from build123d import *

# Parameters (mm, degrees)
SKETCH1_R           = 42.8625
SKETCH1_R_2         = 11.1125
BOSS_EXTRUDE1_DEPTH = 9.525
SKETCH2_R           = 7.9375
CUT_EXTRUDE1_DEPTH  = 10.16
SKETCH3_W           = 3.683
SKETCH3_H           = 25.4
CUT_EXTRUDE2_DEPTH  = 3.429
DRAFT2_ANGLE        = -2.5


with BuildPart() as part:
    # Sketch1 → Boss-Extrude1 (new body, symmetric)
    with BuildSketch(Plane.XY):
        Circle(SKETCH1_R)
        with Locations((0, 24.13)):
            Circle(SKETCH1_R_2, mode=Mode.SUBTRACT)
        with Locations((-20.897192993, -12.065)):
            Circle(SKETCH1_R_2, mode=Mode.SUBTRACT)
        with Locations((20.897192993, -12.065)):
            Circle(SKETCH1_R_2, mode=Mode.SUBTRACT)
    extrude(amount=BOSS_EXTRUDE1_DEPTH, both=True)

    # Sketch2 → Cut-Extrude1 (cut)
    with BuildSketch(Plane.XY.offset(9.525)):
        Circle(SKETCH2_R)
    extrude(amount=-CUT_EXTRUDE1_DEPTH, mode=Mode.SUBTRACT)

    # Sketch3 → Cut-Extrude2 (cut)
    with BuildSketch(Plane.XY.offset(9.525)):
        with Locations((0, -1.27)):
            Rectangle(SKETCH3_W, SKETCH3_H)
    extrude(amount=-CUT_EXTRUDE2_DEPTH, mode=Mode.SUBTRACT)

    # Draft2
    draft2_faces = [part.faces().sort_by_distance(p)[0] for p in [
        (-32.009692993, -12.065, 0),
        (9.784692993, -12.065, 0),
        (-11.1125, 24.13, 0),
    ]]
    draft(draft2_faces, Plane(origin=(0, 0, -9.525), x_dir=(-1, 0, 0), z_dir=(0, 0, -1)), DRAFT2_ANGLE)


solid = part.part
Check sheet for the modelled part. Datum: model origin and axes. Units: mm. A direction names the side the tool comes from. Coordinates: 2 decimals unless noted, no trailing zeros. Loops run counter-clockwise (first coordinate to the right, second up) from the corner with the lowest first, then second, coordinate; pieces in that order, holes last. Notation, with made-up numbers: (70.25, 22.25) -> (99.25, 22.25) arc R21 ccw to (99.25, 58.25) -> close; hole circle Ø9 at (-30.75, -9). An arc over 180 degrees is marked (long way). Answer in a Markdown table with one row per item.
1. Sectioned sample at C-C, the plane x = 0. Record the boundary of the cut face in (y, z) (1 decimal).
Check values:
| item | result |
|---|---|
| outline | (-42.9, -9.5) -> (13, -9.5) -> (12.2, 9.5) -> (11.4, 9.5) -> (11.4, 6.1) -> (7.9, 6.1) -> (7.9, -0.6) -> (-7.9, -0.6) -> (-7.9, 6.1) -> (-14, 6.1) -> (-14, 9.5) -> (-42.9, 9.5) -> close; (35.2, -9.5) -> (42.9, -9.5) -> (42.9, 9.5) -> (36.1, 9.5) -> close |
2. Sectioned sample at B-B, the plane z = 7.25. Record the boundary of the cut face in (x, y) (1 decimal).
Check values:
| item | result |
|---|---|
| outline | circle Ø85.7 at (0, 0); hole circle Ø23.7 at (-20.9, -12.1); hole circle Ø23.7 at (0, 24.1); hole (-1.8, -14) -> (1.8, -14) -> (1.8, -7.7) arc R7.9 ccw to (1.8, 7.7) -> (1.8, 11.4) -> (-1.8, 11.4) -> (-1.8, 7.7) arc R7.9 ccw to (-1.8, -7.7) -> close; hole circle Ø23.7 at (20.9, -12.1) |
3. Sectioned sample at D-D, the plane z = -5.5. Record the boundary of the cut face in (x, y) (1 decimal).
Check values:
| item | result |
|---|---|
| outline | circle Ø85.7 at (0, 0); hole circle Ø22.6 at (-20.9, -12.1); hole circle Ø22.6 at (0, 24.1); hole circle Ø22.6 at (20.9, -12.1) |
4. Access from +Z, -Z, +X, -X, +Y, -Y to the whole of each face (thin tool, end or side, straight path). Record for faces 1 (the face through (-1, 1, -9.525)), 2 (the face through (1.842, 10, 8)).
Check values:
| item | result |
|---|---|
| face 1 | -Z, +X, -X, +Y, -Y |
| face 2 | +Z |
5. Material ranges on line 1 along Y through (x, z) = (0, 6.75); line 2 along Y through (x, z) = (0, 5); line 3 along X through (y, z) = (-13, 0.25), recorded low to high. Write a range as [from, to].
Check values:
| item | result |
|---|---|
| line 1 | y = [-42.86, -13.97], [11.43, 12.31], [35.95, 42.86] |
| line 2 | y = [-42.86, -7.94], [7.94, 12.38], [35.88, 42.86] |
| line 3 | x = [-40.84, -32.4], [-9.4, 9.4], [32.4, 40.84] |
6. Go/stop test with flat-tipped pins: pin 1 (8 mm diameter, centred on x = -30.5, z = -3, fed in from +Y); pin 2 (4 mm diameter, centred on x = -25, z = -2, fed in from -Y); pin 3 (2 mm diameter, centred on x = 33, z = 1.5, fed in from -Y); pin 4 (3 mm diameter, centred on x = 0.5, y = 9.5, fed in from +Z) (3 decimals). Record where each tip stops, or that it passes through.
Check values:
| item | result |
|---|---|
| pin 1 | stops at y = 33.69 |
| pin 2 | stops at y = -36.17 |
| pin 3 | stops at y = -28.52 |
| pin 4 | stops at z = 9.525 |
7. Release check for a two-part mould opening along Y. For faces 3 (the face through (9, 1, 9.525)), 4 (the face through (0, 11.43, 8)), 5 (the face through (23.043, 36.142, 0.133)) record: released by +Y, released by -Y, zero draft, split by the parting line, or undercut.
Check values:
| item | result |
|---|---|
| face 3 | zero draft |
| face 4 | undercut |
| face 5 | split by the parting line |
8. Sectioned sample at A-A, the plane y = 24.13. Record the boundary of the cut face in (x, z) (1 decimal).
Check values:
| item | result |
|---|---|
| outline | (-35.4, -9.5) -> (-11.1, -9.5) -> (-11.9, 9.5) -> (-35.4, 9.5) -> close; (11.1, -9.5) -> (35.4, -9.5) -> (35.4, 9.5) -> (11.9, 9.5) -> close |
